Input: part model. Units: mm. Frame: model coordinates. A direction names the side the tool comes from. Coordinates: 2 decimals unless noted, no trailing zeros. Order: outer loops, then holes, each group sorted by start corner. A loop starts at its lowest first (then second) coordinate and runs counter-clockwise, first axis right, second up. Notation, with made-up numbers: M 43.25,-0.75 L 77.25,-0.75 A4 ccw 77.25,3.25 Z; hole C 62.5,8 d6. An arc over 180 degrees is marked long. Answer in a Markdown table with one row per item.
from build123d import *
from build123d.topology import SkipClean

# Parameters (mm, degrees)
BOSS_EXTRUDE1_DEPTH     = 2
BOSS_EXTRUDE3_START     = 4
BOSS_EXTRUDE3_DEPTH     = 4
CUT_EXTRUDE1_DEPTH      = 22.365860619
SKETCH8_R               = 2.15
CUT_EXTRUDE3_DEPTH      = 4
SKETCH10_R              = 3.1
BOSS_EXTRUDE4_DEPTH     = 1
SKETCH12_R              = 2.4
BOSS_EXTRUDE5_DEPTH     = 7
SKETCH15_R              = 3.1
BOSS_EXTRUDE6_DEPTH     = 1
SKETCH16_R              = 2.15
CUT_EXTRUDE4_DEPTH      = 22.365860619
CUT_EXTRUDE5_DEPTH      = 23.192341021
CUT_EXTRUDE5_DEPTH_BACK = 23.192341021
LPATTERN3_COUNT         = 2
LPATTERN3_PITCH         = 8.02
CUT_EXTRUDE6_DEPTH      = 24.162469696
LPATTERN4_COUNT         = 2
LPATTERN4_PITCH         = 8
CUT_EXTRUDE7_DEPTH      = 24.162469696
FILLET2_R               = 0.5
FILLET3_R               = 0.5


with BuildPart() as part:
    # Sketch2 → Boss-Extrude1 (new, symmetric)
    with BuildSketch(Plane(origin=(0, 0, 0), x_dir=(1, 0, 0), z_dir=(0, 1, 0))):
        with BuildLine():
            Line((0, 3.5), (16, 3.5))
            ThreePointArc((16, 3.5), (19.5, 0), (16, -3.5))
            Line((16, -3.5), (0, -3.5))
            ThreePointArc((0, -3.5), (-3.5, 0), (0, 3.5))
        make_face()
    extrude(amount=BOSS_EXTRUDE1_DEPTH, both=True)

    # Sketch3 → Boss-Extrude3 (add)
    with SkipClean():  # the faces are left unmerged after this step: merging them gives an invalid solid
        with BuildSketch(Plane(origin=(0, 2, 0), x_dir=(1, 0, 0), z_dir=(0, 1, 0)).offset(BOSS_EXTRUDE3_START)):
            with BuildLine():
                Line((1.75, 2.75), (1.75, 2.852630365))
                ThreePointArc((1.75, 2.852630365), (1.705715907, 3.00950412), (1.5859375, 3.120064462))
                ThreePointArc((1.5859375, 3.120064462), (0, 3.5), (-1.5859375, 3.120064462))
                ThreePointArc((-1.5859375, 3.120064462), (-1.705715907, 3.00950412), (-1.75, 2.852630365))
                Line((-1.75, 2.852630365), (-1.75, 2.75))
                ThreePointArc((-1.75, 2.75), (-2.042893219, 2.042893219), (-2.75, 1.75))
                Line((-2.75, 1.75), (-2.852630365, 1.75))
                ThreePointArc((-2.852630365, 1.75), (-3.00950412, 1.705715907), (-3.120064462, 1.5859375))
                ThreePointArc((-3.120064462, 1.5859375), (-3.5, 0), (-3.120064462, -1.5859375))
                ThreePointArc((-3.120064462, -1.5859375), (-3.00950412, -1.705715907), (-2.852630365, -1.75))
                Line((-2.852630365, -1.75), (-2.75, -1.75))
                ThreePointArc((-2.75, -1.75), (-2.042893219, -2.042893219), (-1.75, -2.75))
                Line((-1.75, -2.75), (-1.75, -2.852630365))
                ThreePointArc((-1.75, -2.852630365), (-1.705715907, -3.00950412), (-1.5859375, -3.120064462))
                ThreePointArc((-1.5859375, -3.120064462), (0, -3.5), (1.5859375, -3.120064462))
                ThreePointArc((1.5859375, -3.120064462), (1.705715907, -3.00950412), (1.75, -2.852630365))
                Line((1.75, -2.852630365), (1.75, -2.75))
                ThreePointArc((1.75, -2.75), (2.042893219, -2.042893219), (2.75, -1.75))
                Line((2.75, -1.75), (2.852630365, -1.75))
                ThreePointArc((2.852630365, -1.75), (3.00950412, -1.705715907), (3.120064462, -1.5859375))
                ThreePointArc((3.120064462, -1.5859375), (3.5, 0), (3.120064462, 1.5859375))
                ThreePointArc((3.120064462, 1.5859375), (3.00950412, 1.705715907), (2.852630365, 1.75))
                Line((2.852630365, 1.75), (2.75, 1.75))
                ThreePointArc((2.75, 1.75), (2.042893219, 2.042893219), (1.75, 2.75))
            make_face()
        extrude(amount=-BOSS_EXTRUDE3_DEPTH)

    # Sketch4 → Cut-Extrude1 (cut, through all)
    with SkipClean():  # the faces are left unmerged after this step: merging them gives an invalid solid
        with BuildSketch(Plane(origin=(0, 6, 0), x_dir=(1, 0, 0), z_dir=(0, 1, 0))):
            with BuildLine():
                Line((-0.861545414, -1.212506528), (-0.861545414, -2.150211742))
                ThreePointArc((-0.861545414, -2.150211742), (-0.842839298, -2.208446649), (-0.793719327, -2.244894577))
                ThreePointArc((-0.793719327, -2.244894577), (-0.021545414, -2.372506528), (0.750628499, -2.244894577))
                ThreePointArc((0.750628499, -2.244894577), (0.799748471, -2.208446649), (0.818454586, -2.150211742))
                Line((0.818454586, -2.150211742), (0.818454586, -1.212506528))
                ThreePointArc((0.818454586, -1.212506528), (0.935611874, -0.929663815), (1.218454586, -0.812506528))
                Line((1.218454586, -0.812506528), (2.156159801, -0.812506528))
                ThreePointArc((2.156159801, -0.812506528), (2.214394707, -0.793800412), (2.250842636, -0.744680441))
                ThreePointArc((2.250842636, -0.744680441), (2.378454586, 0.027493472), (2.250842636, 0.799667385))
                ThreePointArc((2.250842636, 0.799667385), (2.214394707, 0.848787357), (2.156159801, 0.867493472))
                Line((2.156159801, 0.867493472), (1.218454586, 0.867493472))
                ThreePointArc((1.218454586, 0.867493472), (0.935611874, 0.98465076), (0.818454586, 1.267493472))
                Line((0.818454586, 1.267493472), (0.818454586, 2.205198686))
                ThreePointArc((0.818454586, 2.205198686), (0.799748471, 2.263433593), (0.750628499, 2.299881522))
                ThreePointArc((0.750628499, 2.299881522), (-0.021545414, 2.427493472), (-0.793719327, 2.299881522))
                ThreePointArc((-0.793719327, 2.299881522), (-0.842839298, 2.263433593), (-0.861545414, 2.205198686))
                Line((-0.861545414, 2.205198686), (-0.861545414, 1.267493472))
                ThreePointArc((-0.861545414, 1.267493472), (-0.978702701, 0.98465076), (-1.261545414, 0.867493472))
                Line((-1.261545414, 0.867493472), (-2.199250628, 0.867493472))
                ThreePointArc((-2.199250628, 0.867493472), (-2.257485535, 0.848787357), (-2.293933463, 0.799667385))
                ThreePointArc((-2.293933463, 0.799667385), (-2.421545414, 0.027493472), (-2.293933463, -0.744680441))
                ThreePointArc((-2.293933463, -0.744680441), (-2.257485535, -0.793800412), (-2.199250628, -0.812506528))
                Line((-2.199250628, -0.812506528), (-1.261545414, -0.812506528))
                ThreePointArc((-1.261545414, -0.812506528), (-0.978702701, -0.929663815), (-0.861545414, -1.212506528))
            make_face()
        cut_extrude1 = extrude(amount=-CUT_EXTRUDE1_DEPTH, mode=Mode.SUBTRACT)

    # Sketch8 → Cut-Extrude3 (cut)
    with SkipClean():  # the faces are left unmerged after this step: merging them gives an invalid solid
        with BuildSketch(Plane(origin=(0, 2, 0), x_dir=(1, 0, 0), z_dir=(0, 1, 0))):
            with Locations(Location((16, 0, 0), (0, 0, 270))):
                Circle(SKETCH8_R)
        extrude(amount=-CUT_EXTRUDE3_DEPTH, mode=Mode.SUBTRACT)

    # Sketch10 → Boss-Extrude4 (add)
    with SkipClean():  # the faces are left unmerged after this step: merging them gives an invalid solid
        with BuildSketch(Plane(origin=(0, -2, 0), x_dir=(-1, 0, 0), z_dir=(0, -1, 0))):
            with Locations(Location((-16, 0, 0), (0, 0, 270))):
                Circle(SKETCH10_R)
        extrude(amount=BOSS_EXTRUDE4_DEPTH)

    # Sketch12 → Boss-Extrude5 (add)
    with SkipClean():  # the faces are left unmerged after this step: merging them gives an invalid solid
        with BuildSketch(Plane(origin=(0, -2, 0), x_dir=(-1, 0, 0), z_dir=(0, -1, 0))):
            with Locations(Location((-16, 0, 0), (0, 0, 90))):
                Circle(SKETCH12_R)
        extrude(amount=BOSS_EXTRUDE5_DEPTH)

    # Sketch15 → Boss-Extrude6 (add)
    with SkipClean():  # the faces are left unmerged after this step: merging them gives an invalid solid
        with BuildSketch(Plane(origin=(0, -9, 0), x_dir=(-1, 0, 0), z_dir=(0, -1, 0))):
            with Locations(Location((-16, 0, 0), (0, 0, 270))):
                Circle(SKETCH15_R)
        extrude(amount=BOSS_EXTRUDE6_DEPTH)

    # Sketch16 → Cut-Extrude4 (cut, through all)
    with SkipClean():  # the faces are left unmerged after this step: merging them gives an invalid solid
        with BuildSketch(Plane(origin=(0, -2, 0), x_dir=(1, 0, 0), z_dir=(0, 1, 0))):
            with Locations(Location((16, 0, 0), (0, 0, 270))):
                Circle(SKETCH16_R)
        extrude(amount=-CUT_EXTRUDE4_DEPTH, mode=Mode.SUBTRACT)

    # Sketch17 → Cut-Extrude5 (cut, two sides: drawn at the far end of the back side and taken through both)
    with SkipClean():  # the faces are left unmerged after this step: merging them gives an invalid solid
        with BuildSketch(Plane(origin=(0, 0, 0), x_dir=(0, 0, -1), z_dir=(1, 0, 0)).offset(-CUT_EXTRUDE5_DEPTH_BACK)):
            with BuildLine():
                Line((-0.5, -10), (-0.5, -8))
                ThreePointArc((-0.5, -8), (0, -7.5), (0.5, -8))
                Line((0.5, -8), (0.5, -10))
                ThreePointArc((0.5, -10), (0, -10.5), (-0.5, -10))
            make_face()
        extrude(amount=CUT_EXTRUDE5_DEPTH + CUT_EXTRUDE5_DEPTH_BACK, mode=Mode.SUBTRACT)

    # LPattern3: Cut-Extrude1 ×2
    with SkipClean():  # the faces are left unmerged after this step: merging them gives an invalid solid
        with Locations(*[(i * LPATTERN3_PITCH, 0, 0) for i in range(1, LPATTERN3_COUNT)]):
            add(cut_extrude1, mode=Mode.SUBTRACT)

    # Sketch20 → Cut-Extrude6 (cut, through all)
    with SkipClean():  # the faces are left unmerged after this step: merging them gives an invalid solid
        with BuildSketch(Plane(origin=(0, 2, 0), x_dir=(1, 0, 0), z_dir=(0, 1, 0))):
            with BuildLine():
                Line((11.330011313, 2.427493472), (12.668443274, 2.427493472))
                ThreePointArc((12.668443274, 2.427493472), (13.017140291, 2.223479161), (13.010141399, 1.819545424))
                ThreePointArc((13.010141399, 1.819545424), (12.500118007, 0.028740879), (12.98066258, -1.770198166))
                ThreePointArc((12.98066258, -1.770198166), (12.982671335, -2.171348997), (12.635595447, -2.372506528))
                Line((12.635595447, -2.372506528), (11.362859139, -2.372506528))
                ThreePointArc((11.362859139, -2.372506528), (11.015783251, -2.171348997), (11.017792006, -1.770198166))
                ThreePointArc((11.017792006, -1.770198166), (11.498336579, 0.028740879), (10.988313187, 1.819545424))
                ThreePointArc((10.988313187, 1.819545424), (10.981314296, 2.223479161), (11.330011313, 2.427493472))
            make_face()
        cut_extrude6 = extrude(amount=-CUT_EXTRUDE6_DEPTH, mode=Mode.SUBTRACT)

    # LPattern4: Cut-Extrude6 ×2
    with Locations(*[(-i * LPATTERN4_PITCH, 0, 0) for i in range(1, LPATTERN4_COUNT)]):
        add(cut_extrude6, mode=Mode.SUBTRACT)

    # Sketch25 → Cut-Extrude7 (cut, through all)
    with BuildSketch(Plane(origin=(0, 2, 0), x_dir=(1, 0, 0), z_dir=(0, 1, 0))):
        with BuildLine():
            Line((16, 3.5), (16, 3.1))
            ThreePointArc((16, 3.1), (19.1, 0), (16, -3.1))
            Line((16, -3.1), (16, -3.5))
            ThreePointArc((16, -3.5), (19.5, 0), (16, 3.5))
        make_face()
    extrude(amount=-CUT_EXTRUDE7_DEPTH, mode=Mode.SUBTRACT)

    # Fillet2
    # the kernel refuses this fillet: 0.5 mm, written as the material it adds along each edge
    with BuildSketch(Plane(origin=(16, 2, 3.1), x_dir=(0.9976162063830436, 0, -0.06900655593423367), z_dir=(0, -1, 0))) as fillet2_piece_1:
        with BuildLine():
            CenterArc((0.462343925, 0.498808103), FILLET2_R, 191.509080872, 74.533990047)
            Line((-0.027602622, 0.399046483), (-0.037401553, 0.39705125))
            ThreePointArc((-0.037401553, 0.39705125), (-0.023777473, 0.198833176), (-0.009976162, -0.000690066))
            Line((-0.009976162, -0.000690066), (0.000690066, -0.009976162))
            ThreePointArc((0.000690066, -0.009976162), (0.213920323, -0.00261024), (0.427150581, -0.009976162))
            Line((0.427150581, -0.009976162), (0.427840647, 0))
        make_face()
    extrude(amount=4)

    # Fillet3
    # the kernel refuses this fillet: 0.5 mm, written as the material it adds along each edge
    with BuildSketch(Plane(origin=(16, 2, -3.1), x_dir=(0, 0, -1), z_dir=(0, -1, 0))) as fillet3_piece_1:
        with BuildLine():
            CenterArc((0.465714286, 0.495662822), FILLET3_R, 187.913858162, 74.533990047)
            Line((-0.02952381, 0.426820763), (-0.039428571, 0.425443922))
            ThreePointArc((-0.039428571, 0.425443922), (-0.017365922, 0.213230258), (-0.01, 0))
            Line((-0.01, 0), (0, -0.01))
            ThreePointArc((0, -0.01), (0.2, -0.01), (0.398685714, -0.009913256))
            Line((0.398685714, -0.009913256), (0.4, 0))
        make_face()
    extrude(amount=4)


solid = part.part
1) Mould query, pull axis X, two halves, no side actions, for faces 1 (the face through (8.838, 0, 2)), 2 (the face through (2.051, 4.028, -2.035)), 3 (the face through (-0.862, 2, 2)), 4 (the face through (7, -2, 2)). Classes: +X half, -X half, draft (parallel to the pull), parting line (faces both ways), or undercut.
Resolved:
| item | result |
|---|---|
| face 1 | undercut |
| face 2 | +X half |
| face 3 | undercut |
| face 4 | draft |
2) Cut plane B-B, the plane z = 0. State how many separate pieces and enclosed holes the cut face has, and give its area (3 significant figures).
Resolved:
| item | result |
|---|---|
| separate pieces | 6 |
| enclosed holes | 0 |
| area | 39.7 mm2 |
3) Cut plane D-D, the plane y = -8.25. Output: boundary loops of the cut face in (x, z).
Resolved:
| item | result |
|---|---|
| outline | M 13.65,-0.5 A2.4 ccw 18.35,-0.5 L 18.09,-0.5 A2.15 cw 13.91,-0.5 Z; M 13.65,0.5 L 13.91,0.5 A2.15 cw 18.09,0.5 L 18.35,0.5 A2.4 ccw Z |
4) Contact query for flat-ended pins moving along their axis: pin 1 (0.8 mm diameter, centred on x = -2, z = 2.5, fed in from +Y); pin 2 (1 mm diameter, centred on x = 10.5, z = -0.5, fed in from -Y); pin 3 (0.5 mm diameter, centred on x = -1.5, y = 1.5, fed in from +Z); pin 4 (1.3 mm diameter, centred on x = 16.5, z = -1.5, fed in from +Y). Output: stop coordinate, or through.
Resolved:
| item | result |
|---|---|
| pin 1 | stops at y = 6 |
| pin 2 | stops at y = -2 |
| pin 3 | stops at z = 3.27 |
| pin 4 | stops at y = 2 |
5) Reachability of faces 5 (the face through (18.5, -9.4, -0.5)), 6 (the face through (15.8, -9, 2.6)), 7 (the face through (18, -3, 2)), 8 (the face through (-2.42, 2.06, -0.04)), 9 (the face through (16, -9, -2.6)) from +Z, -Z, +X, -X, +Y, -Y: full face, straight path, thin tool, end or side. Return the list, or none.
Resolved:
| item | result |
|---|---|
| face 5 | +X, -X, -Y |
| face 6 | +Z |
| face 7 | none |
| face 8 | +Y, -Y |
| face 9 | -Z |
6) Material intervals for probe 1 along Z at (x, y) = (0.75, 1.5); probe 2 along Y at (x, z) = (14.5, 2); probe 3 along X at (y, z) = (-5.5, 0), sorted ascending.
Resolved:
| item | result |
|---|---|
| probe 1 | z = -3.5 to -2.3, 2.25 to 3.5 |
| probe 2 | y = -10 to -9, -3 to 2 |
| probe 3 | x = 13.6 to 13.85, 18.15 to 18.4 |
7) Cut plane A-A, the plane x = 6.5. Output: boundary loops of the cut face in (y, z), and give its area (3 significant figures).
Resolved:
| item | result |
|---|---|
| outline | M -2,-3.5 L 2,-3.5 L 2,-0.87 L -2,-0.87 Z; M -2,0.81 L 2,0.81 L 2,3.5 L -2,3.5 Z |
| area | 21.3 mm2 |
8) Cut plane C-C, the plane y = -6. Output: boundary loops of the cut face in (x, z), and give its area (3 significant figures).
Resolved:
| item | result |
|---|---|
| outline | C 16,0 d4.8; hole C 16,0 d4.3 |
| area | 3.57 mm2 |
